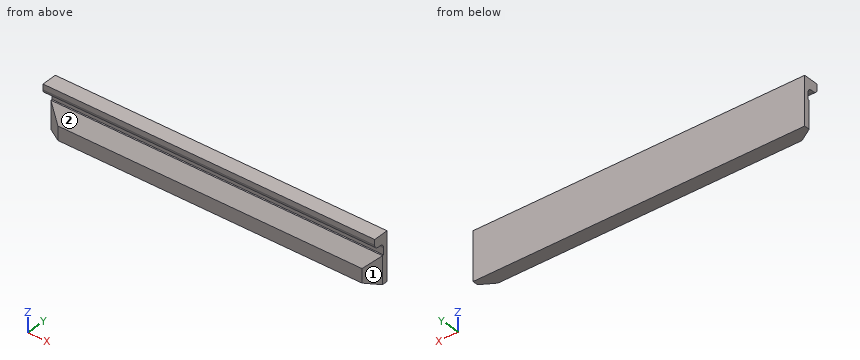
from build123d import *

# Parameters (mm, degrees)
SKETCH1_W           = 240
SKETCH1_H           = 35
BOSS_EXTRUDE1_DEPTH = 3
SKETCH3_W           = 240
SKETCH3_H           = 7
BOSS_EXTRUDE3_DEPTH = 8
FILLET1_R           = 3
SKETCH4_W           = 240
SKETCH4_H           = 7
BOSS_EXTRUDE5_DEPTH = 20
CHAMFER1_SIZE       = 10
CHAMFER1_SIZE2      = 6


with BuildPart() as part:
    # Sketch1 → Boss-Extrude1 (new body)
    with BuildSketch(Plane(origin=(0, 0, 0), x_dir=(1, 0, 0), z_dir=(0, 1, 0))):
        Rectangle(SKETCH1_W, SKETCH1_H)
    extrude(amount=BOSS_EXTRUDE1_DEPTH)

    # Sketch3 → Boss-Extrude3 (add)
    with BuildSketch(Plane.XZ):
        with Locations((0, 14)):
            Rectangle(SKETCH3_W, SKETCH3_H)
    extrude(amount=BOSS_EXTRUDE3_DEPTH)

    # Fillet1
    fillet1_edges = [part.edges().sort_by_distance(p)[0] for p in [
        (0, 0, 10.5),
        (0, -8, 10.5),
    ]]
    fillet(fillet1_edges, radius=FILLET1_R)

    # Sketch4 → Boss-Extrude5 (add)
    with BuildSketch(Plane(origin=(0, 0, -17.5), x_dir=(-1, 0, 0), z_dir=(0, 0, -1))):
        with Locations((0, -3.5)):
            Rectangle(SKETCH4_W, SKETCH4_H)
    extrude(amount=-BOSS_EXTRUDE5_DEPTH)

    # Chamfer1
    chamfer1_edges = [part.edges().sort_by_distance(p)[0] for p in [
        (0, -7, 2.5),
        (-120, -7, -7.5),
        (120, -7, -7.5),
    ]]
    chamfer1_side = [part.faces().sort_by_distance(p)[0] for p in [
        (0, -7, -7.5),
    ]]
    chamfer(chamfer1_edges, length=CHAMFER1_SIZE, length2=CHAMFER1_SIZE2, reference=chamfer1_side[0])


solid = part.part
The listing builds one solid part. Answer for the finished solid, in the listing's coordinates (mm). Face numbers are marked on the shaded views. Give positions to 0.01 mm unless a question says otherwise; leave off trailing zeros. Order: outer loops, then holes, each group sorted by start corner. A loop starts at its lowest first (then second) coordinate and runs counter-clockwise, first axis right, second up. Notation, with made-up numbers: (-13, 71) - (13, 71) arc R21 cw to (13, 92) - close; hole circle Ø2 at (42, 42.25). An arc over 180 degrees is marked (long way). Use one line per item in the form item = value.
1) Each of these flat-tipped pins is pushed along its axis until it touches: pin 1 (5 mm diameter, centred on y = -3, z = -7.5, fed in from +X); pin 2 (12 mm diameter, centred on x = 83.5, z = -0.5, fed in from -Y); pin 3 (3 mm diameter, centred on x = 21, z = -14.5, fed in from -Y); pin 4 (2.5 mm diameter, centred on x = -17, z = 5.5, fed in from -Y). Where does it stop, or does it pass through?
Verdict:
pin_1 = 120
pin_2 = -6.4
pin_3 = -7
pin_4 = 0
2) The mould has two halves that part along Z. Classify the marked faces 1 and 2: released by +Z, released by -Z, zero draft, split by the parting line, or undercut.
Verdict:
face_1 = zero draft
face_2 = undercut
3) Consider probe 1 along Z at (x, y) = (-67, -4.5); probe 2 along Y at (x, z) = (-33.5, -15); probe 3 along Z at (x, y) = (87, -0.5). Determine where each line is inside the solid, lowest interval first. Write a range as [from, to].
Verdict:
probe_1 = [-17.5, -3.33], [10.5, 17.5]
probe_2 = [-7, 3]
probe_3 = [-17.5, 2.5], [9.16, 17.5]
4) Find section B-B on z = -15. Determine the outline of the cut face in (x, y).
Verdict:
outline = (-120, -1) - (-110, -7) - (110, -7) - (120, -1) - (120, 3) - (-120, 3) - close
5) Find section A-A on x = 55. Determine the outline of the cut face in (y, z).
Verdict:
outline = (-8, 13.5) arc R3 ccw to (-5, 10.5) - (-3, 10.5) arc R3 cw to (0, 7.5) - (0, 2.5) - (-1, 2.5) - (-7, -7.5) - (-7, -17.5) - (3, -17.5) - (3, 17.5) - (-8, 17.5) - close
6) Find section C-C on z = 5. Determine the outline of the cut face in (x, y), and give its area (3 significant figures).
Verdict:
outline = (-120, 0) - (120, 0) - (120, 3) - (-120, 3) - close
area = 720 mm^2
